Work out the finished part from the listing and answer in its coordinate system (mm). Face numbers are marked on the shaded views. A direction names the side the tool comes from. Round coordinates to 2 decimals unless told otherwise and drop trailing zeros. Loops run counter-clockwise (first coordinate to the right, second up) from the corner with the lowest first, then second, coordinate; pieces in that order, holes last. Notation, with made-up numbers: (20, 8) - (47, 8) arc R32 ccw to (47, 43) - close; hole circle Ø10 at (1.25, -34.75). An arc over 180 degrees is marked (long way). Answer as CSV lines item,"result". Start each with the question number.
Q1. Section A-A on x = -10 is taken. Write down the section's boundary in (y, z), then the cut area to 3 significant figures.
Q2. The mould has two halves that part along X. Classify the marked faces 4, 5 and 6: +X half, -X half, draft (parallel to the pull), parting line (faces both ways), or undercut.
Q3. Straight lines are drawn through the part: L1, parallel to Y at x = 9, z = 40; L2, parallel to X at y = -6, z = 41; L3, parallel to Y at x = 12.5, z = 20. For each, find the intervals that lie inside material, in ascending order. Write a range as [from, to].
Q4. Section B-B on z = 29 is taken. Write down the section's boundary in (x, y), then the cut area to 3 significant figures.
Q5. For the marked faces 1, 2 and 3, determine the directions among +Z, -Z, +X, -X, +Y, -Y from which every point of the face is accessible in a straight line to the end or side of a thin tool.
Q6. Section D-D on y = -2 is taken. Write down the section's boundary in (x, z).
Q7. Each of these flat-tipped pins is pushed along its axis until it touches: pin 1 Ø8 at (x, y) = (-10, -8) entering from +Z; pin 2 Ø1.8 at (x, z) = (-17, 41.5) entering from -Y; pin 3 Ø8 at (y, z) = (-9, 32.5) entering from +X. Where does it stop, or does it pass through?
Q8. Section C-C on z = 41.5 is taken. Write down the section's boundary in (x, y).
```python
from build123d import *

# Parameters (mm, degrees)
EXTRUDE_1_DEPTH = 50
SKETCH_2_R      = 3
EXTRUDE_2_DEPTH = 10


with BuildPart() as part:
    # 草图1 → 凸台-拉伸1 (new body)
    with BuildSketch(Plane.XY):
        with BuildLine():
            Line((-48.193457488, 66.287565891), (11.806542512, 66.287565891))
            ThreePointArc((11.806542512, 66.287565891), (15.342076418, 64.823099797), (16.806542512, 61.287565891))
            Line((16.806542512, 61.287565891), (16.806542512, 1.287565891))
            ThreePointArc((16.806542512, 1.287565891), (15.342076418, -2.247968015), (11.806542512, -3.712434109))
            Line((11.806542512, -3.712434109), (-48.193457488, -3.712434109))
            ThreePointArc((-48.193457488, -3.712434109), (-51.728991394, -2.247968015), (-53.193457488, 1.287565891))
            Line((-53.193457488, 1.287565891), (-53.193457488, 61.287565891))
            ThreePointArc((-53.193457488, 61.287565891), (-51.728991394, 64.823099797), (-48.193457488, 66.287565891))
        make_face()
    extrude(amount=EXTRUDE_1_DEPTH)

    # 草图2 → 凸台-拉伸2 (add)
    with BuildSketch(Plane.XZ.offset(3.712434109)):
        with BuildLine():
            Line((-18.193457488, 9), (-35.193457488, 9))
            ThreePointArc((-35.193457488, 9), (-37.314777832, 9.878679656), (-38.193457488, 12))
            Line((-38.193457488, 12), (-38.193457488, 46))
            ThreePointArc((-38.193457488, 46), (-37.314777832, 48.121320344), (-35.193457488, 49))
            Line((-35.193457488, 49), (-1.193457488, 49))
            ThreePointArc((-1.193457488, 49), (0.927862855, 48.121320344), (1.806542512, 46))
            Line((1.806542512, 46), (1.806542512, 12))
            ThreePointArc((1.806542512, 12), (0.927862855, 9.878679656), (-1.193457488, 9))
            Line((-1.193457488, 9), (-18.193457488, 9))
        make_face()
        with Locations((-18.193457488, 41.5)):
            Circle(SKETCH_2_R, mode=Mode.SUBTRACT)
        with Locations((-30.693457488, 29)):
            Circle(SKETCH_2_R, mode=Mode.SUBTRACT)
        with Locations((-18.193457488, 16.5)):
            Circle(SKETCH_2_R, mode=Mode.SUBTRACT)
        with Locations((-5.693457488, 29)):
            Circle(SKETCH_2_R, mode=Mode.SUBTRACT)
    extrude(amount=EXTRUDE_2_DEPTH)


solid = part.part
```
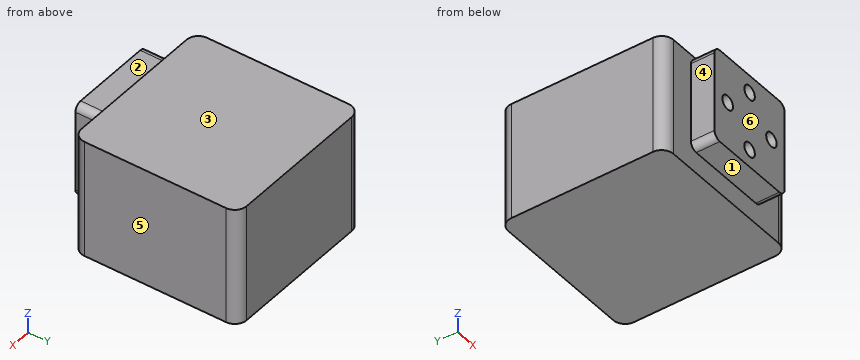
Findings:
1,outline,"(-13.71, 9) - (-3.71, 9) - (-3.71, 0) - (66.29, 0) - (66.29, 50) - (-3.71, 50) - (-3.71, 49) - (-13.71, 49) - close"
1,area,"3,900 mm^2"
2,face 4,"-X half"
2,face 5,"+X half"
2,face 6,"draft"
3,L1,"y = [-3.71, 66.29]"
3,L2,"x = [-38.19, -21.15], [-15.24, 1.81]"
3,L3,"y = [-3.66, 66.24]"
4,outline,"(-53.19, 1.29) arc R5 ccw to (-48.19, -3.71) - (-38.19, -3.71) - (-38.19, -13.71) - (-33.69, -13.71) - (-33.69, -3.71) - (-27.69, -3.71) - (-27.69, -13.71) - (-8.69, -13.71) - (-8.69, -3.71) - (-2.69, -3.71) - (-2.69, -13.71) - (1.81, -13.71) - (1.81, -3.71) - (11.81, -3.71) arc R5 ccw to (16.81, 1.29) - (16.81, 61.29) arc R5 ccw to (11.81, 66.29) - (-48.19, 66.29) arc R5 ccw to (-53.19, 61.29) - close"
4,area,"5,160 mm^2"
5,face 1,"-Z, +X, -X, -Y"
5,face 2,"+Z, +X, -X, -Y"
5,face 3,"+Z, +X, -X, +Y, -Y"
6,outline,"(-51.96, 0) - (15.57, 0) - (15.57, 50) - (-51.96, 50) - close"
7,pin 1,"stops at z = 49"
7,pin 2,"stops at y = -3.71"
7,pin 3,"stops at x = 1.81"
8,outline,"(-53.19, 1.29) arc R5 ccw to (-48.19, -3.71) - (-38.19, -3.71) - (-38.19, -13.71) - (-21.19, -13.71) - (-21.19, -3.71) - (-15.19, -3.71) - (-15.19, -13.71) - (1.81, -13.71) - (1.81, -3.71) - (11.81, -3.71) arc R5 ccw to (16.81, 1.29) - (16.81, 61.29) arc R5 ccw to (11.81, 66.29) - (-48.19, 66.29) arc R5 ccw to (-53.19, 61.29) - close"
